from build123d import *

# Parameters (mm, degrees)
SKETCH1_R           = 12.7
SKETCH1_R_2         = 3.302
BOSS_EXTRUDE1_DEPTH = 9.525


with BuildPart() as part:
    # Sketch1 → Boss-Extrude1 (new body)
    with BuildSketch(Plane(origin=(0, 0, 0), x_dir=(1, 0, 0), z_dir=(0, 1, 0))):
        with BuildLine():
            Line((7.62, 22.86), (7.62, 18.272118104))
            ThreePointArc((7.62, 18.272118104), (7.813305115, 17.598598895), (8.334375, 17.130110722))
            ThreePointArc((8.334375, 17.130110722), (19.05, 0), (8.334375, -17.130110722))
            ThreePointArc((8.334375, -17.130110722), (7.813305115, -17.598598895), (7.62, -18.272118104))
            Line((7.62, -18.272118104), (7.62, -22.86))
            ThreePointArc((7.62, -22.86), (0, -30.48), (-7.62, -22.86))
            Line((-7.62, -22.86), (-7.62, -18.272118104))
            ThreePointArc((-7.62, -18.272118104), (-7.813305115, -17.598598895), (-8.334375, -17.130110722))
            ThreePointArc((-8.334375, -17.130110722), (-19.05, 0), (-8.334375, 17.130110722))
            ThreePointArc((-8.334375, 17.130110722), (-7.813305115, 17.598598895), (-7.62, 18.272118104))
            Line((-7.62, 18.272118104), (-7.62, 22.86))
            ThreePointArc((-7.62, 22.86), (0, 30.48), (7.62, 22.86))
        make_face()
        Circle(SKETCH1_R, mode=Mode.SUBTRACT)
        with Locations((0, 22.86)):
            Circle(SKETCH1_R_2, mode=Mode.SUBTRACT)
        with Locations((0, -22.86)):
            Circle(SKETCH1_R_2, mode=Mode.SUBTRACT)
    extrude(amount=BOSS_EXTRUDE1_DEPTH)


solid = part.part
Can you work these out from the model? Positions are in its coordinate system, mm. A direction names the side the tool comes from. Give positions to 0.01 mm unless a question says otherwise; leave off trailing zeros. Order: outer loops, then holes, each group sorted by start corner. A loop starts at its lowest first (then second) coordinate and runs counter-clockwise, first axis right, second up. Notation, with made-up numbers: M 77,41.5 L 125,41.5 A34 cw 125,71.5 Z; hole C 87,71 d9. An arc over 180 degrees is marked long. One line per question, with ' | ' between items.
Item 1: Suppose I cut it at C-C, the plane z = -4.5. Write out the boundary of the cut face in (x, y) (3 decimals), then the cut area to 3 significant figures.
Answer block:
outline: M -18.511,0 L -11.876,0 L -11.876,9.525 L -18.511,9.525 Z; M 11.876,0 L 18.511,0 L 18.511,9.525 L 11.876,9.525 Z | area: 126 mm2
Item 2: Suppose I cut it at A-A, the plane x = 0. Write out the boundary of the cut face in (y, z) (3 decimals), then the cut area to 3 significant figures.
Answer block:
outline: M 0,-30.48 L 9.525,-30.48 L 9.525,-26.162 L 0,-26.162 Z; M 0,-19.558 L 9.525,-19.558 L 9.525,-12.7 L 0,-12.7 Z; M 0,12.7 L 9.525,12.7 L 9.525,19.558 L 0,19.558 Z; M 0,26.162 L 9.525,26.162 L 9.525,30.48 L 0,30.48 Z | area: 213 mm2
Item 3: I'm going to push flat-ended pins straight in: pin 1 Ø3 at (y, z) = (7, -1.5) entering from +X; pin 2 Ø3.5 at (y, z) = (4.5, 20.5) entering from -X; pin 3 Ø1.4 at (y, z) = (2.5, 21.5) entering from +X. Where does each tip first touch, or does it pass through?
Answer block:
pin 1: stops at x = 19.05 | pin 2: stops at x = -7.62 | pin 3: stops at x = 7.62
Item 4: Please list where these lines run through material, in increasing order: L1, parallel to Z at x = 0, y = 2; L2, parallel to X at y = 2.5, z = -22.86; L3, parallel to X at y = 7, z = 0.
Answer block:
L1: z = -30.48 to -26.16, -19.56 to -12.7, 12.7 to 19.56, 26.16 to 30.48 | L2: x = -7.62 to -3.3, 3.3 to 7.62 | L3: x = -19.05 to -12.7, 12.7 to 19.05
Item 5: We'd pull the mould along X, two halves only. Please class faces 6 (the face through (-7.62, 5, 21)), 7 (the face through (7.82, 4.7, 17.59)), 8 (the face through (1.52, 4.7, -19.93)), 9 (the face through (-0.17, 4.7, -30.48)): released by +X, released by -X, zero draft, split by the parting line, or undercut.
Answer block:
face 6: released by -X | face 7: released by +X | face 8: undercut | face 9: split by the parting line
Item 6: Suppose I cut it at B-B, the plane y = 2.75. Write out the boundary of the cut face in (x, z).
Answer block:
outline: M -8.33,-17.13 A1.27 cw -7.62,-18.27 L -7.62,-22.86 A7.62 ccw 7.62,-22.86 L 7.62,-18.27 A1.27 cw 8.33,-17.13 A19.05 ccw 8.33,17.13 A1.27 cw 7.62,18.27 L 7.62,22.86 A7.62 ccw -7.62,22.86 L -7.62,18.27 A1.27 cw -8.33,17.13 A19.05 ccw Z; hole C 0,0 d25.4; hole C 0,-22.86 d6.6; hole C 0,22.86 d6.6
Item 7: For faces 1 (the face through (-7.62, 5, -21)), 2 (the face through (7.62, 5, -21)), 3 (the face through (-2.75, 4.7, 12.4)), 4 (the face through (0.17, 4.7, 30.48)), 5 (the face through (7.62, 5, 21)), which set-ups out of +Z, -Z, +X, -X, +Y, -Y let a thin tool reach every point of the face, with its end or its side?
Answer block:
face 1: -Z, -X, +Y, -Y | face 2: -Z, +X, +Y, -Y | face 3: +Y, -Y | face 4: +Z, +Y, -Y | face 5: +Z, +X, +Y, -Y
Item 8: Suppose I cut it at D-D, the plane x = -4. Write out the boundary of the cut face in (y, z) (3 decimals), then the cut area to 3 significant figures.
Answer block:
outline: M 0,-29.346 L 9.525,-29.346 L 9.525,-12.054 L 0,-12.054 Z; M 0,12.054 L 9.525,12.054 L 9.525,29.346 L 0,29.346 Z | area: 329 mm2
